Check sheet for the drawn part. Datum: minimum x, y, z corner. Units: mm. A direction names the side the tool comes from. Coordinates: 2 decimals unless noted, no trailing zeros. Order: outer loops, then holes, each group sorted by start corner. A loop starts at its lowest first (then second) coordinate and runs counter-clockwise, first axis right, second up.
Q1. Cross-section at C-C, the plane y = 6.25. Record the boundary of the cut face in (x, z), and give its area (3 significant figures).
Q2. Cross-section at B-B, the plane z = 8.03. Record the boundary of the cut face in (x, y), and give its area (3 significant figures).
Q3. Cross-section at D-D, the plane z = 5.5. Record the boundary of the cut face in (x, y).
Q4. Set-up check for the marked faces 4 and 5: record each of +Z, -Z, +X, -X, +Y, -Y from which the full face is reachable in a straight line by a thin tool's end or side.
Q5. Thickness scan on line 1 (Z direction, x = 31, y = 6.55); line 2 (Z direction, x = 13.5, y = 1); line 3 (X direction, y = 6, z = 8.25). Record the ranges inside material, lowest first.
Q6. Depth check by flat-ended pin: P1, Ø2, axis at x = 15.6, z = 8.03, coming from the -Y side (1 decimal); P2, Ø1, axis at x = 18.5, z = 10.5, coming from the -Y side. Enter the tip coordinate at first touch or a pass-through.
Q7. Draft check along X on the marked faces 1, 2 and 3. Enter one of: pulls with the +X half, pulls with the -X half, needs draft (parallel to the pull), parting line crosses it, or undercut.
Q8. Cross-section at A-A, the plane x = 31. Record the boundary of the cut face in (y, z), and give its area (3 significant figures).
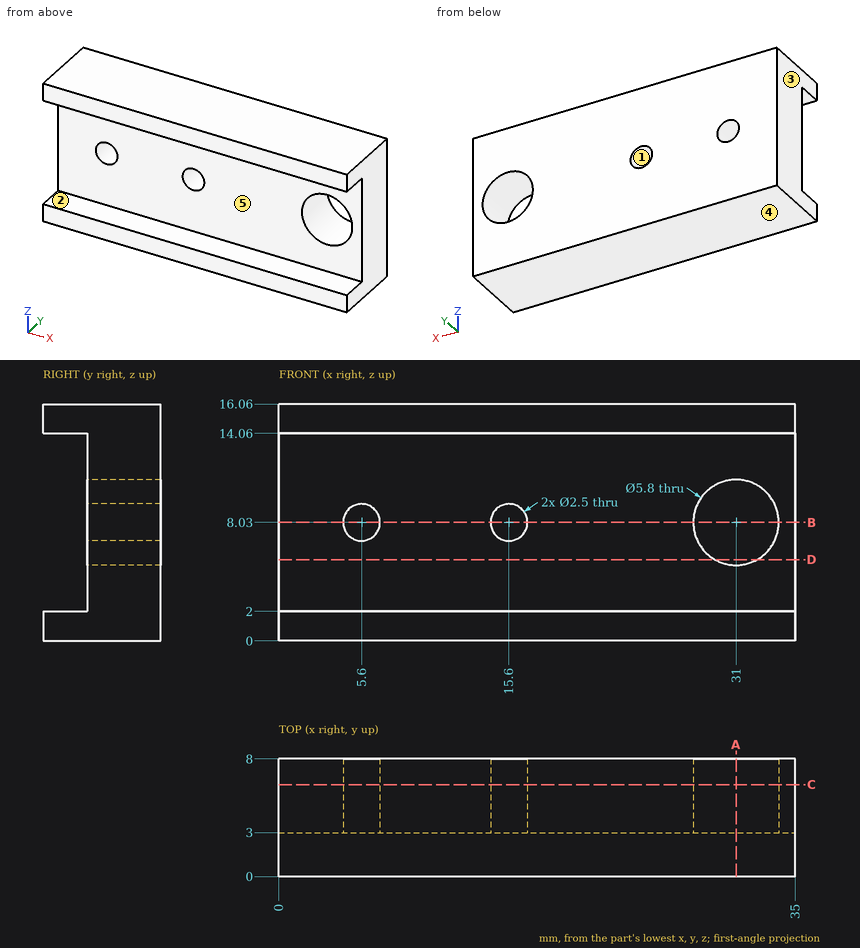
Check values:
1. outline: (0, 0) - (35, 0) - (35, 16.06) - (0, 16.06) - close; hole circle Ø2.5 at (5.6, 8.03); hole circle Ø2.5 at (15.6, 8.03); hole circle Ø5.8 at (31, 8.03)
1. area: 526 mm2
2. outline: (0, 3) - (4.35, 3) - (4.35, 8) - (0, 8) - close; (6.85, 3) - (14.35, 3) - (14.35, 8) - (6.85, 8) - close; (16.85, 3) - (28.1, 3) - (28.1, 8) - (16.85, 8) - close; (33.9, 3) - (35, 3) - (35, 8) - (33.9, 8) - close
2. area: 121 mm2
3. outline: (0, 3) - (29.58, 3) - (29.58, 8) - (0, 8) - close; (32.42, 3) - (35, 3) - (35, 8) - (32.42, 8) - close
4. face 4: -Z, +X, -X, +Y, -Y
4. face 5: +X, -X, -Y
5. line 1: z = 0 to 5.13, 10.93 to 16.06
5. line 2: z = 0 to 2, 14.06 to 16.06
5. line 3: x = 0 to 4.37, 6.83 to 14.37, 16.83 to 28.11, 33.89 to 35
6. P1: passes through
6. P2: stops at y = 3
7. face 1: undercut
7. face 2: needs draft
7. face 3: pulls with the -X half
8. outline: (0, 0) - (8, 0) - (8, 5.13) - (3, 5.13) - (3, 2) - (0, 2) - close; (0, 14.06) - (3, 14.06) - (3, 10.93) - (8, 10.93) - (8, 16.06) - (0, 16.06) - close
8. area: 63.3 mm2
